Verification items for this drawing (mm, ordinates from the low corner). A direction names the side the tool comes from. Round coordinates to 2 decimals unless told otherwise and drop trailing zeros. Write each loop counter-clockwise with the first axis right and the second up, starting at its lowest first coordinate (ties: lowest second). Pieces come first, ordered by that corner, then holes.
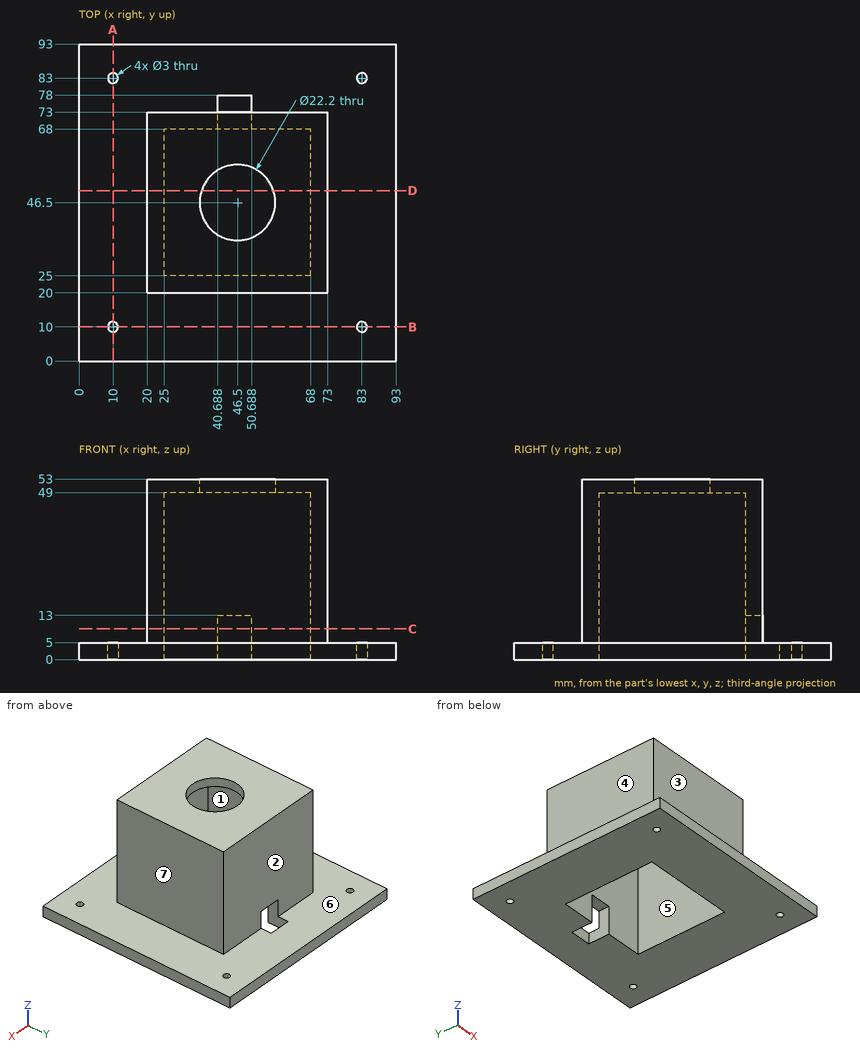
1. Section check A-A (x = 10). Record the cut outline in (y, z).
2. Access from +Z, -Z, +X, -X, +Y, -Y to the whole of each face (thin tool, end or side, straight path). Record for the marked faces 1, 2, 3 and 4.
3. Depth check by flat-ended pin: pin 1 Ø5 at (x, y) = (11.5, 52.5) entering from +Z; pin 2 Ø13 at (y, z) = (39, 25.5) entering from -X; pin 3 Ø13 at (x, z) = (50, 13) entering from +Y; pin 4 Ø8 at (x, y) = (51, 47) entering from -Z. Enter the tip coordinate at first touch or a pass-through.
4. Scan lines: line 1 along Y through (x, z) = (10, 3); line 2 along X through (y, z) = (44, 38). Record each from-to range of solid material in increasing order.
5. Section check D-D (y = 50). Record the cut outline in (x, z).
6. Release check for a two-part mould opening along X. For the marked faces 5, 6 and 7 record: +X half, -X half, draft (parallel to the pull), parting line (faces both ways), or undercut.
7. Section check C-C (z = 9). Record the cut outline in (x, y), plus the area to 3 significant figures.
Results below:
1. outline: (0, 0) - (8.5, 0) - (8.5, 5) - (0, 5) - close; (11.5, 0) - (81.5, 0) - (81.5, 5) - (11.5, 5) - close; (84.5, 0) - (93, 0) - (93, 5) - (84.5, 5) - close
2. face 1: -Z
2. face 2: +Z, +X, -X, +Y
2. face 3: +Z, +X, -X, -Y
2. face 4: +Z, -X, +Y, -Y
3. pin 1: stops at z = 5
3. pin 2: stops at x = 20
3. pin 3: stops at y = 73
3. pin 4: passes through
4. line 1: y = 0 to 8.5, 11.5 to 81.5, 84.5 to 93
4. line 2: x = 20 to 25, 68 to 73
5. outline: (0, 0) - (25, 0) - (25, 49) - (35.97, 49) - (35.97, 53) - (20, 53) - (20, 5) - (0, 5) - close; (57.03, 49) - (68, 49) - (68, 0) - (93, 0) - (93, 5) - (73, 5) - (73, 53) - (57.03, 53) - close
6. face 5: undercut
6. face 6: draft
6. face 7: +X half
7. outline: (20, 20) - (73, 20) - (73, 73) - (50.69, 73) - (50.69, 68) - (68, 68) - (68, 25) - (25, 25) - (25, 68) - (40.69, 68) - (40.69, 73) - (20, 73) - close
7. area: 910 mm2
